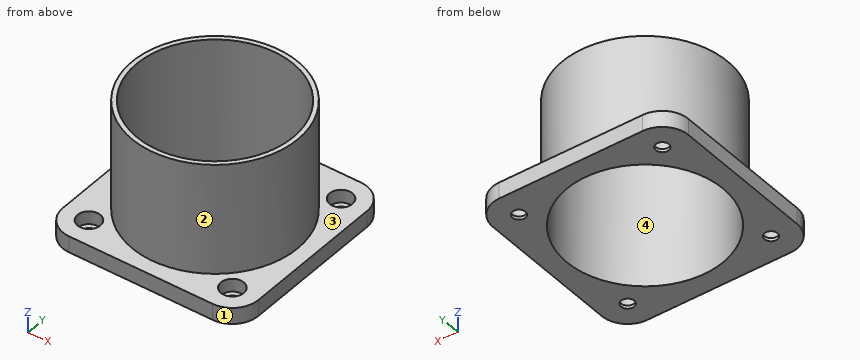
from build123d import *

# Parameters (mm, degrees)
F0_R           = 24
F1_DEPTH       = 5
F2_R           = 25.4
F2_R_2         = 24
F3_DEPTH       = 34
F4_D           = 4
F4_CBORE_D     = 7
F4_CBORE_DEPTH = 4


with BuildPart() as f1:
    # F0 (on Top) → F1 (new body)
    with BuildSketch(Plane.XY):
        with BuildLine():
            Line((22, 30), (-22, 30))
            ThreePointArc((-22, 30), (-27.656854, 27.656854), (-30, 22))
            Line((-30, 22), (-30, -22))
            ThreePointArc((-30, -22), (-27.656854, -27.656854), (-22, -30))
            Line((-22, -30), (22, -30))
            ThreePointArc((22, -30), (27.656854, -27.656854), (30, -22))
            Line((30, -22), (30, 22))
            ThreePointArc((30, 22), (27.656854, 27.656854), (22, 30))
        make_face()
        Circle(F0_R, mode=Mode.SUBTRACT)
    extrude(amount=-F1_DEPTH)

    # F2 (on face) → F3 (join)
    with BuildSketch(Plane.XY):
        Circle(F2_R)
        Circle(F2_R_2, mode=Mode.SUBTRACT)
    extrude(amount=F3_DEPTH)

    # F4 (through all)
    with Locations(Plane.XY):
        with Locations((-22, -22), (22, -22), (22, 22), (-22, 22)):
            CounterBoreHole(F4_D / 2, F4_CBORE_D / 2, F4_CBORE_DEPTH)


solid = f1.part
Source: CAD feature listing. Evaluate the final solid. Frame: model axes, mm. Face numbers are marked on the shaded views. Give positions to 0.01 mm unless a question says otherwise; leave off trailing zeros. Write each loop counter-clockwise with the first axis right and the second up, starting at its lowest first coordinate (ties: lowest second). Pieces come first, ordered by that corner, then holes. Notation, with made-up numbers: M 58.5,52.25 L 105.5,52.25 A31 ccw 105.5,87.25 Z; hole C 37.5,18 d10. An arc over 180 degrees is marked long. Answer as a JSON object with one key per item and string values.
Q1. Ray query, line 1 along Y through (x, z) = (22, -1); line 2 along Y through (x, z) = (20.5, -1.5); line 3 along Z through (x, y) = (-25, -23). Return the intervals inside material, ascending.
Geometry check:
{"line 1": "y = -30 to -25.5, -18.5 to -9.59, 9.59 to 18.5, 25.5 to 30", "line 2": "y = -30 to -25.16, -18.84 to -12.48, 12.48 to 18.84, 25.16 to 30", "line 3": "z = -5 to -4"}
Q2. Cut plane A-A, the plane y = 0. Return the cut outline in (x, z), then the cut area to 3 significant figures.
Geometry check:
{"outline": "M -30,-5 L -24,-5 L -24,34 L -25.4,34 L -25.4,0 L -30,0 Z; M 24,-5 L 30,-5 L 30,0 L 25.4,0 L 25.4,34 L 24,34 Z", "area": "155 mm^2"}
Q3. Contact query for flat-ended pins moving along their axis: P1, Ø2, axis at x = -21.5, y = 21, coming from the +Z side; P2, Ø2, axis at y = -18, z = 15.5, coming from the +X side; P3, Ø9, axis at x = 22, y = -22, coming from the +Z side. Output: stop coordinate, or through.
Geometry check:
{"P1": "stops at z = -4", "P2": "stops at x = 18.87", "P3": "stops at z = 0"}
Q4. Cut plane C-C, the plane z = 21. Return the cut outline in (x, y), then the cut area to 3 significant figures.
Geometry check:
{"outline": "C 0,0 d50.8; hole C 0,0 d48", "area": "217 mm^2"}
Q5. Mould query, pull axis X, two halves, no side actions, for the marked faces 1, 2, 3 and 4. Classes: +X half, -X half, draft (parallel to the pull), parting line (faces both ways), or undercut.
Geometry check:
{"face 1": "+X half", "face 2": "parting line", "face 3": "draft", "face 4": "undercut"}
